Build history of the part. All positions in model axes, mm. Face numbers are marked on the shaded views. A direction names the side the tool comes from. Coordinates: 2 decimals unless noted, no trailing zeros. Order: outer loops, then holes, each group sorted by start corner. A loop starts at its lowest first (then second) coordinate and runs counter-clockwise, first axis right, second up. Notation, with made-up numbers: (-36.75, 65.5) - (18.25, 65.5) arc R31 cw to (18.25, 97.5) - close; hole circle Ø7 at (33, 81.5). An arc over 180 degrees is marked (long way). One line per item, written item: value.
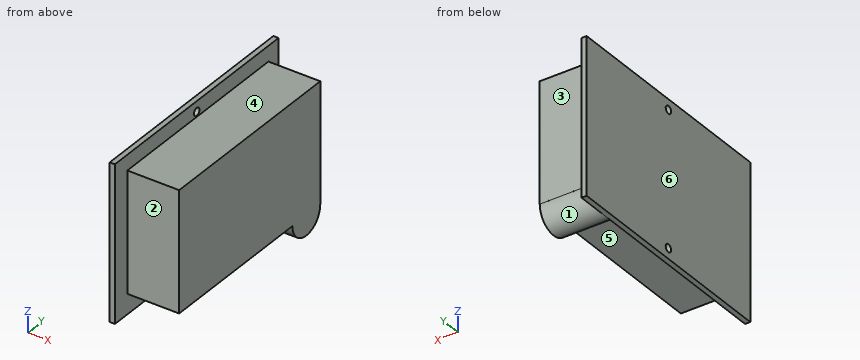
from build123d import *

# Parameters (mm, degrees)
F0_W     = 45
F0_H     = 30
F0_R     = 0.75
F1_DEPTH = 1
F3_DEPTH = 10


with BuildPart() as f1:
    # F0 (on Right) → F1 (new body)
    with BuildSketch(Plane.YZ):
        with Locations((22.5, 15)):
            Rectangle(F0_W, F0_H)
        with Locations((22.5, 2)):
            Circle(F0_R, mode=Mode.SUBTRACT)
        with Locations((22.5, 28)):
            Circle(F0_R, mode=Mode.SUBTRACT)
    extrude(amount=F1_DEPTH)

    # F2 (on face) → F3 (join)
    with BuildSketch(Plane.YZ.offset(1)):
        with BuildLine():
            Line((42.216498, 27.034795), (3.409794, 27.034795))
            Line((3.409794, 27.034795), (3.409794, 3.871003))
            Line((3.409794, 3.871003), (34.534011, 3.871003))
            ThreePointArc((34.534011, 3.871003), (38.41285, 0.07055), (42.213303, 3.949389))
            Line((42.213303, 3.949389), (42.216498, 3.949389))
            Line((42.216498, 3.949389), (42.216498, 27.034795))
        make_face()
    extrude(amount=F3_DEPTH)


solid = f1.part
1. 3-axis set-ups, long thin cutter, end or side, ignore diameter. For the marked faces 5 and 6: which of +Z, -Z, +X, -X, +Y, -Y reach the whole face in a straight line?
Values found:
face 5: -Z, +X, -Y
face 6: +Z, -Z, -X, +Y, -Y
2. Band-saw the part on A-A, the plane y = 22.5. Give the cut face in (x, z).
Values found:
outline: (0, 0) - (1, 0) - (1, 1.25) - (0, 1.25) - close; (0, 2.75) - (1, 2.75) - (1, 3.87) - (11, 3.87) - (11, 27.03) - (1, 27.03) - (1, 27.25) - (0, 27.25) - close; (0, 28.75) - (1, 28.75) - (1, 30) - (0, 30) - close
3. Flat gauge pins, fed straight in: P1, Ø1, axis at x = 6.5, y = 7, coming from the +Z side; P2, Ø1.2, axis at y = 22.5, z = 2, coming from the -X side; P3, Ø5, axis at x = 7.5, z = 17, coming from the -Y side; P4, Ø5, axis at x = 7.5, z = 19.5, coming from the +Y side. Where does each tip first touch, or does it go through?
Values found:
P1: stops at z = 27.03
P2: passes through
P3: stops at y = 3.41
P4: stops at y = 42.22
4. Probe line 1 along Z through (x, y) = (0.35, 22.5); line 2 along Z through (x, y) = (5.5, 9); line 3 along X through (y, z) = (3, 8.75). List the from-to ranges inside material, lowest first.
Values found:
line 1: z = 0 to 1.25, 2.75 to 27.25, 28.75 to 30
line 2: z = 3.87 to 27.03
line 3: x = 0 to 1
5. Two-plate mould, pull along Y, no slides. Class the marked faces 1, 2, 3 and 4: pulls with the +Y half, pulls with the -Y half, needs draft (parallel to the pull), parting line crosses it, or undercut.
Values found:
face 1: parting line crosses it
face 2: pulls with the -Y half
face 3: pulls with the +Y half
face 4: needs draft
6. Band-saw the part on B-B, the plane z = 2. Give the cut face in (x, y), and give its area (3 significant figures).
Values found:
outline: (0, 0) - (1, 0) - (1, 21.75) - (0, 21.75) - close; (0, 23.25) - (1, 23.25) - (1, 35.04) - (11, 35.04) - (11, 41.7) - (1, 41.7) - (1, 45) - (0, 45) - close
area: 110 mm2
7. Band-saw the part on D-D, the plane y = 7. Give the cut face in (x, z), and give its area (3 significant figures).
Values found:
outline: (0, 0) - (1, 0) - (1, 3.87) - (11, 3.87) - (11, 27.03) - (1, 27.03) - (1, 30) - (0, 30) - close
area: 262 mm2
